from build123d import *

# Parameters (mm, degrees)
F0_W     = 60
F0_H     = 30
F1_DEPTH = 30
F2_W     = 30
F2_H     = 30
F3_DEPTH = 30
F3_TAPER = 10
F4_R     = 6.8497431599
F5_DEPTH = 25.4


with BuildPart() as f1:
    # F0 (on Front) → F1 (new body)
    with BuildSketch(Plane.XZ):
        with Locations((0.4317071289, 0.4612154852)):
            Rectangle(F0_W, F0_H)
    extrude(amount=F1_DEPTH)

    # F2 (on face) → F3 (join)
    with BuildSketch(Plane.XY.offset(15.4612154852)):
        with Locations((15.4317071289, -15)):
            Rectangle(F2_W, F2_H)
    extrude(amount=F3_DEPTH, taper=F3_TAPER)

    # F4 (on face) → F5 (cut)
    with BuildSketch(Plane.XY.offset(45.4612154852)):
        with Locations((15.4317071289, -15)):
            Circle(F4_R)
    extrude(amount=-F5_DEPTH, mode=Mode.SUBTRACT)


solid = f1.part
Could you check a few things on this model? Use its own coordinates, in mm. A direction names the side the tool comes from. Give positions to 0.01 mm unless a question says otherwise; leave off trailing zeros. Loops run counter-clockwise (first coordinate to the right, second up) from the corner with the lowest first, then second, coordinate; pieces in that order, holes last. Notation, with made-up numbers: M -1,36 L 55,36 A16 cw 55,56 Z; hole C 88,-20.5 d4. An arc over 180 degrees is marked long. Answer as a JSON object with one key per item and string values.
Q1. If I drill on probe 1 along Z at (x, y) = (-1, -25.25); probe 2 along Y at (x, z) = (20, 39); probe 3 along X at (y, z) = (-9.75, 40), over which ranges is the centre line in solid material (lowest first)? Write a range as [from, to].
Values found:
{"probe 1": "z = [-14.54, 15.46]", "probe 2": "y = [-25.85, -20.1], [-9.9, -4.15]", "probe 3": "x = [4.76, 11.03], [19.83, 26.1]"}
Q2. Suppose I cut it at B-B, the plane z = 22.5. List the corners of the cut face in (x, y) for me.
Values found:
{"outline": "M 1.67,-28.76 L 29.19,-28.76 L 29.19,-1.24 L 1.67,-1.24 Z; hole C 15.43,-15 d13.7"}
Q3. Suppose I cut it at A-A, the plane y = -15. List the corners of the cut face in (x, z) for me.
Values found:
{"outline": "M -29.57,-14.54 L 30.43,-14.54 L 30.43,15.46 L 25.14,45.46 L 22.28,45.46 L 22.28,20.06 L 8.58,20.06 L 8.58,45.46 L 5.72,45.46 L 0.43,15.46 L -29.57,15.46 Z"}
Q4. For P1, Ø12, axis at y = -24, z = 27.5, coming from the -X side; P2, Ø2, axis at x = 0, z = 17.5, coming from the -Y side; P3, Ø5, axis at x = -10, y = -7.5, coming from the +Z side, each with a flat end and sliding along its axis, tell me the tip position at first contact or that it passes through.
Values found:
{"P1": "stops at x = 1.5", "P2": "stops at y = -29.77", "P3": "stops at z = 15.46"}
Q5. If we mould it in two halves opening along Y, with no side actions, what happens to faces 3 (the flat face through (15, -15, 20.061)), 4 (the flat face through (15.642, -27.392, 30.251)), 5 (the flat face through (-15, -15, 15.461))? For each: pulls with the +Y half, pulls with the -Y half, needs draft (parallel to the pull), parting line crosses it, or undercut.
Values found:
{"face 3": "undercut", "face 4": "pulls with the -Y half", "face 5": "needs draft"}
Q6. For faces 1 (the flat face through (8.8, -12.7, 45.461)), 2 (the cylindrical face through (21.965, -12.943, 32.939)), which set-ups out of +Z, -Z, +X, -X, +Y, -Y let a thin tool reach every point of the face, with its end or its side?
Values found:
{"face 1": "+Z, +X, -X, +Y, -Y", "face 2": "+Z"}
Q7. Suppose I cut it at D-D, the plane y = -19.75. List the corners of the cut face in (x, z) for me.
Values found:
{"outline": "M -29.57,-14.54 L 30.43,-14.54 L 30.43,15.46 L 25.14,45.46 L 20.37,45.46 L 20.37,20.06 L 10.5,20.06 L 10.5,45.46 L 5.72,45.46 L 0.43,15.46 L -29.57,15.46 Z"}
Q8. Suppose I cut it at C-C, the plane x = 6.5. List the corners of the cut face in (y, z) for me.
Values found:
{"outline": "M -30,-14.54 L 0,-14.54 L 0,15.46 L -5.29,45.46 L -24.71,45.46 L -30,15.46 Z"}
